```python
from build123d import *

# Parameters (mm, degrees)
SKETCH2_W                               = 45
SKETCH2_H                               = 20
BOSS_EXTRUDE2_DEPTH                     = 14.16787265
FILLET1_R                               = 10
CUT_EXTRUDE1_DEPTH                      = 22
CBORE_FOR_M5_HEX_HEAD_BOLT1_D           = 5.5
CBORE_FOR_M5_HEX_HEAD_BOLT1_CBORE_D     = 12
CBORE_FOR_M5_HEX_HEAD_BOLT1_CBORE_DEPTH = 10
FILLET2_R                               = 3


with BuildPart() as part:
    # Sketch2 → Boss-Extrude2 (new body)
    with BuildSketch(Plane.XY):
        Rectangle(SKETCH2_W, SKETCH2_H)
    extrude(amount=BOSS_EXTRUDE2_DEPTH)

    # Fillet1
    fillet1_edges = [part.edges().sort_by_distance(p)[0] for p in [
        (22.5, 10, 7.083936325),
        (22.5, -10, 7.083936325),
        (-22.5, 10, 7.083936325),
        (-22.5, -10, 7.083936325),
    ]]
    fillet(fillet1_edges, radius=FILLET1_R - 0.0001)  # a hair under: the kernel refuses the full size

    # Sketch3 → Cut-Extrude1 (cut)
    with BuildSketch(Plane.XZ.offset(10)):
        with BuildLine():
            Line((-4, 0), (-4, 3))
            ThreePointArc((-4, 3), (0, 7), (4, 3))
            Line((4, 3), (4, 0))
            ThreePointArc((4, 0), (0, -4), (-4, 0))
        make_face()
    extrude(amount=-CUT_EXTRUDE1_DEPTH, mode=Mode.SUBTRACT)

    # CBORE for M5 Hex Head Bolt1 (through all)
    with Locations(Plane.XY.offset(14.16787265)):
        with Locations((-12.5, 0), (12.5, 0)):
            CounterBoreHole(CBORE_FOR_M5_HEX_HEAD_BOLT1_D / 2, CBORE_FOR_M5_HEX_HEAD_BOLT1_CBORE_D / 2, CBORE_FOR_M5_HEX_HEAD_BOLT1_CBORE_DEPTH)

    # Fillet2
    fillet2_edges = [part.edges().sort_by_distance(p)[0] for p in [
        (0, 10, 14.16787265),
        (0, -10, 14.16787265),
        (-19.571097101, -7.071097101, 14.16787265),
        (-19.571097101, 7.071097101, 14.16787265),
        (19.571097101, -7.071097101, 14.16787265),
        (19.571097101, 7.071097101, 14.16787265),
    ]]
    fillet(fillet2_edges, radius=FILLET2_R)


solid = part.part
```
Design review of the part built by this model. Coordinates are the model's own, in mm. A direction names the side the tool comes from. Give positions to 0.01 mm unless a question says otherwise; leave off trailing zeros. Loops run counter-clockwise (first coordinate to the right, second up) from the corner with the lowest first, then second, coordinate; pieces in that order, holes last. Notation, with made-up numbers: M -33.75,-37.5 L -27.75,-37.5 A3 ccw -27.75,-32.5 Z; hole C -13.75,-2.5 d8. An arc over 180 degrees is marked long. Return JSON: item names as keys, results as strings. Group by question number.
Item 1: We need section C-C (x = 0). Give the boundary of the cut face in (y, z).
Item 2: We need section A-A (z = 2). Give the number of separate pieces and of enclosed holes in the cut face, and give its area (3 significant figures).
Item 3: We need section D-D (x = -8.5). Give the boundary of the cut face in (y, z).
Item 4: Tool access review of faces 5 (the flat face through (0, 10, 8)), 6 (the flat face through (4, 0, 2)), 7 (the cylindrical face through (-6.777, 1.802, 9.238)): name each direction out of +Z, -Z, +X, -X, +Y, -Y from which nothing blocks a thin tool from reaching the whole face with its end or side.
Item 5: For probe 1 along Y at (x, z) = (12.5, 6.25); probe 2 along X at (y, z) = (-0.25, 1.75); probe 3 along Y at (x, z) = (12.5, 2.5), list the stretches that pass through material, from the lowest coordinate up.
Item 6: Insertion check: pin 1 Ø2 at (x, z) = (-8.5, 12.5) entering from +Y; pin 2 Ø6.5 at (x, y) = (-12.5, 0) entering from +Z; pin 3 Ø5 at (x, z) = (-16.5, 9) entering from -Y. Each pin has a flat end and moves straight along its axis. Give the tip position at first contact, or say it passes through.
Item 7: Mouldability with a two-part tool opening along Y and no side actions: class faces 1 (the cylindrical face through (-19.65, -6.99, 5.66)), 2 (the flat face through (-11, -3, 4.168)), 3 (the flat face through (-4, 0, 1)), 4 (the flat face through (14, -3, 4.168)) as released by +Y, released by -Y, zero draft, split by the parting line, or undercut.
Output:
{
 "1": {"outline": "M -10,7 L 10,7 L 10,11.17 A3 ccw 7,14.17 L -7,14.17 A3 ccw -10,11.17 Z"},
 "2": {"separate pieces": "2", "enclosed holes": "2", "area": "607 mm^2"},
 "3": {"outline": "M -10,0 L 10,0 L 10,11.17 A3 ccw 7,14.17 L 4.47,14.17 L 4.47,4.17 L -4.47,4.17 L -4.47,14.17 L -7,14.17 A3 ccw -10,11.17 Z"},
 "4": {"face 5": "+Z, -Z, +X, -X, +Y", "face 6": "-Z, +Y, -Y", "face 7": "+Z"},
 "5": {"probe 1": "y = -10 to -6, 6 to 10", "probe 2": "x = -22.5 to -15.24, -9.76 to -4, 4 to 9.76, 15.24 to 22.5", "probe 3": "y = -10 to -2.75, 2.75 to 10"},
 "6": {"pin 1": "stops at y = 9.98", "pin 2": "stops at z = 4.17", "pin 3": "stops at y = -9.89"},
 "7": {"face 1": "released by -Y", "face 2": "undercut", "face 3": "zero draft", "face 4": "undercut"}
}
